from build123d import *

# Parameters (mm, degrees)
F0_W     = 67.47918
F0_H     = 143.993221
F1_DEPTH = 12.7
F2_R     = 12.7
F3_R     = 25.4
F4_DEPTH = 12.7
F5_R     = 3.592793
F6_DEPTH = 12.7
F7_R     = 24.765
F8_DEPTH = 12.7


with BuildPart() as f1:
    # F0 (on Top) → F1 (new body, symmetric)
    with BuildSketch(Plane.XY):
        with Locations((-37.244237, -1.34131)):
            Rectangle(F0_W, F0_H)
    extrude(amount=F1_DEPTH, both=True)

    # F2
    f2_edges = [f1.edges().sort_by_distance(p)[0] for p in [
        (-70.983827, -73.33792, 0),
        (-3.504647, -73.33792, 0),
        (-3.504647, 70.655301, 0),
        (-70.983827, 70.655301, 0),
    ]]
    fillet(f2_edges, radius=F2_R)

    # F3 (on face) → F4 (cut)
    with BuildSketch(Plane.XY.offset(12.7)):
        with Locations((-37.201827, -32.69792)):
            Circle(F3_R)
    extrude(amount=-F4_DEPTH, mode=Mode.SUBTRACT)

    # F5 (on face) → F6 (cut, through all)
    with BuildSketch(Plane.XY):
        with Locations((-37.201827, -32.69792)):
            Circle(F5_R)
    extrude(amount=-F6_DEPTH, mode=Mode.SUBTRACT)

    # F7 (on face) → F8 (join)
    with BuildSketch(Plane.XY.offset(12.7)):
        with Locations((-37.304053, 30.650346)):
            Circle(F7_R)
    extrude(amount=F8_DEPTH)


solid = f1.part
Source: CAD feature listing. Evaluate the final solid. Frame: model axes, mm. A direction names the side the tool comes from. Coordinates: 2 decimals unless noted, no trailing zeros. Loops run counter-clockwise (first coordinate to the right, second up) from the corner with the lowest first, then second, coordinate; pieces in that order, holes last. Notation, with made-up numbers: (-33, -19) -> (18, -19) arc R23 cw to (18, -2) -> close; hole circle Ø8 at (5, -8.75). An arc over 180 degrees is marked (long way). Answer in a Markdown table with one row per item. Add a question column.
Q1. Section D-D on x = -48. Return the cut outline in (y, z).
Q2. Section B-B on x = -29. Return the cut outline in (y, z), and give its area (3 significant figures).
Q3. Section A-A on z = 2.5. Return the cut outline in (x, y), and give its area (3 significant figures).
Q4. Ray query, line 1 along Z through (x, y) = (-10, 61.5); line 2 along Y through (x, z) = (-29, 1.5); line 3 along Z through (x, y) = (-34.5, -21). Return the intervals inside material, ascending.
Q5. Pull-direction query (X, two-part tool) for faces 1 (the face through (-38, 0, -12.7)), 2 (the face through (-14.427, 21.165, 18.961)), 3 (the face through (-35.27, -29.67, -6.26)); classes: pulls with the +X half, pulls with the -X half, needs draft (parallel to the pull), parting line crosses it, or undercut.
Q6. Reachability of faces 4 (the face through (-32, -32, 0)), 5 (the face through (-38, 31, 25.4)) from +Z, -Z, +X, -X, +Y, -Y: full face, straight path, thin tool, end or side. Return the list, or none.
Q7. Section C-C on y = 22.5. Return the cut outline in (x, z).
Q8. Contact query for flat-ended pins moving along their axis: pin 1 Ø6 at (x, z) = (-59.5, 5) entering from -Y; pin 2 Ø10 at (x, z) = (-36, 20) entering from -Y; pin 3 Ø1.5 at (x, y) = (-53, -6.5) entering from +Z. Output: stop coordinate, or through.
Computed values:
| question | item | result |
|---|---|---|
| 1 | outline | (-73.34, -12.7) -> (70.66, -12.7) -> (70.66, 12.7) -> (52.99, 12.7) -> (52.99, 25.4) -> (8.31, 25.4) -> (8.31, 12.7) -> (-9.71, 12.7) -> (-9.71, 0) -> (-55.69, 0) -> (-55.69, 12.7) -> (-73.34, 12.7) -> close |
| 2 | outline | (-73.34, -12.7) -> (70.66, -12.7) -> (70.66, 12.7) -> (53.98, 12.7) -> (53.98, 25.4) -> (7.32, 25.4) -> (7.32, 12.7) -> (-8.66, 12.7) -> (-8.66, 0) -> (-56.74, 0) -> (-56.74, 12.7) -> (-73.34, 12.7) -> close |
| 2 | area | 3,640 mm^2 |
| 3 | outline | (-70.98, -60.64) arc R12.7 ccw to (-58.28, -73.34) -> (-16.2, -73.34) arc R12.7 ccw to (-3.5, -60.64) -> (-3.5, 57.96) arc R12.7 ccw to (-16.2, 70.66) -> (-58.28, 70.66) arc R12.7 ccw to (-70.98, 57.96) -> close; hole circle Ø50.8 at (-37.2, -32.7) |
| 3 | area | 7,550 mm^2 |
| 4 | line 1 | z = -12.7 to 12.7 |
| 4 | line 2 | y = -73.34 to -56.74, -8.66 to 70.66 |
| 4 | line 3 | z = -12.7 to 0 |
| 5 | face 1 | needs draft |
| 5 | face 2 | parting line crosses it |
| 5 | face 3 | undercut |
| 6 | face 4 | +Z |
| 6 | face 5 | +Z, +X, -X, +Y, -Y |
| 7 | outline | (-70.98, -12.7) -> (-3.5, -12.7) -> (-3.5, 12.7) -> (-13.92, 12.7) -> (-13.92, 25.4) -> (-60.69, 25.4) -> (-60.69, 12.7) -> (-70.98, 12.7) -> close |
| 8 | pin 1 | stops at y = -73.34 |
| 8 | pin 2 | stops at y = 5.89 |
| 8 | pin 3 | stops at z = 12.7 |
